from build123d import *

# Parameters (mm, degrees)
F1_DEPTH       = 22.86
F3_DEPTH       = 23.368
F5_DEPTH       = 45.72
F7_D           = 4.9784
F7_START       = 6.6163719
F7_CBORE_D     = 9.652
F7_CBORE_DEPTH = 2.54
F9_D           = 4.9784
F9_DEPTH       = 31.75
F9_CBORE_D     = 9.652
F9_CBORE_DEPTH = 12.7
F9_TIP         = 1.4956622529


with BuildPart() as f1:
    # F0 (on Front) → F1 (new body, symmetric)
    with BuildSketch(Plane.XZ):
        with BuildLine():
            ThreePointArc((-38.7916133821, 0), (-20.5036133821, 18.288), (-2.2156133821, 0))
            Line((-2.2156133821, 0), (10.4843866179, 0))
            Line((10.4843866179, 0), (26.3593866179, 0))
            Line((26.3593866179, 0), (42.2343866179, 0))
            Line((42.2343866179, 0), (49.8543866179, 0))
            Line((49.8543866179, 0), (49.8543866179, 19.05))
            Line((49.8543866179, 19.05), (-0.1977932308, 19.05))
            ThreePointArc((-0.1977932308, 19.05), (-3.2353429752, 19.6542062107), (-5.8104533064, 21.3748399243))
            Line((-5.8104533064, 21.3748399243), (-9.8356133821, 25.4))
            Line((-9.8356133821, 25.4), (-31.1716133821, 25.4))
            Line((-31.1716133821, 25.4), (-43.8716133821, 12.7))
            Line((-43.8716133821, 12.7), (-43.8716133821, 0))
            Line((-43.8716133821, 0), (-38.7916133821, 0))
        make_face()
        with BuildLine():
            ThreePointArc((-21.3164133821, -18.2699288493), (-33.7194264558, -12.640934649), (-38.7916133821, 0))
            Line((-38.7916133821, 0), (-43.8716133821, 0))
            Line((-43.8716133821, 0), (-43.8716133821, -12.7))
            Line((-43.8716133821, -12.7), (-31.1716133821, -25.4))
            Line((-31.1716133821, -25.4), (-21.3164133821, -25.4))
            Line((-21.3164133821, -25.4), (-21.3164133821, -18.2699288493))
        make_face()
        with BuildLine():
            ThreePointArc((-38.7916133821, 0), (-20.5036133821, 18.288), (-2.2156133821, 0))
            Line((-2.2156133821, 0), (10.4843866179, 0))
            Line((10.4843866179, 0), (26.3593866179, 0))
            Line((26.3593866179, 0), (42.2343866179, 0))
            Line((42.2343866179, 0), (49.8543866179, 0))
            Line((49.8543866179, 0), (49.8543866179, 19.05))
            Line((49.8543866179, 19.05), (-0.1977932308, 19.05))
            ThreePointArc((-0.1977932308, 19.05), (-3.2353429752, 19.6542062107), (-5.8104533064, 21.3748399243))
            Line((-5.8104533064, 21.3748399243), (-9.8356133821, 25.4))
            Line((-9.8356133821, 25.4), (-31.1716133821, 25.4))
            Line((-31.1716133821, 25.4), (-43.8716133821, 12.7))
            Line((-43.8716133821, 12.7), (-43.8716133821, 0))
            Line((-43.8716133821, 0), (-38.7916133821, 0))
        make_face()
        with BuildLine():
            Line((10.4843866179, 0), (-2.2156133821, 0))
            ThreePointArc((-2.2156133821, 0), (-7.2878003084, -12.640934649), (-19.6908133821, -18.2699288493))
            Line((-19.6908133821, -18.2699288493), (-19.6908133821, -25.4))
            Line((-19.6908133821, -25.4), (-9.8356133821, -25.4))
            Line((-9.8356133821, -25.4), (-5.8104533064, -21.3748399243))
            ThreePointArc((-5.8104533064, -21.3748399243), (-3.2353429752, -19.6542062107), (-0.1977932308, -19.05))
            Line((-0.1977932308, -19.05), (49.8543866179, -19.05))
            Line((49.8543866179, -19.05), (49.8543866179, 0))
            Line((49.8543866179, 0), (42.2343866179, 0))
            Line((42.2343866179, 0), (26.3593866179, 0))
            Line((26.3593866179, 0), (10.4843866179, 0))
        make_face()
    extrude(amount=F1_DEPTH, both=True)

    # F2 (on Top) → F3 (cut, symmetric)
    with BuildSketch(Plane.XY):
        with BuildLine():
            ThreePointArc((42.2135652835, -0.8128), (42.2291804306, -0.4065333221), (42.2343866179, 0))
            ThreePointArc((42.2343866179, 0), (42.2291804306, 0.4065333221), (42.2135652835, 0.8128))
            ThreePointArc((42.2135652835, 0.8128), (25.9528532958, 15.8697938127), (10.4843866179, 0))
            ThreePointArc((10.4843866179, 0), (25.9528532958, -15.8697938127), (42.2135652835, -0.8128))
        make_face()
        with BuildLine():
            ThreePointArc((42.2135652835, -0.8128), (42.2291804306, -0.4065333221), (42.2343866179, 0))
            ThreePointArc((42.2343866179, 0), (42.2291804306, 0.4065333221), (42.2135652835, 0.8128))
            ThreePointArc((42.2135652835, 0.8128), (25.9528532958, 15.8697938127), (10.4843866179, 0))
            ThreePointArc((10.4843866179, 0), (25.9528532958, -15.8697938127), (42.2135652835, -0.8128))
        make_face()
        with BuildLine():
            ThreePointArc((42.2135652835, 0.8128), (42.2291804306, 0.4065333221), (42.2343866179, 0))
            ThreePointArc((42.2343866179, 0), (42.2291804306, -0.4065333221), (42.2135652835, -0.8128))
            Line((42.2135652835, -0.8128), (49.8543866179, -0.8128))
            Line((49.8543866179, -0.8128), (49.8543866179, 0.8128))
            Line((49.8543866179, 0.8128), (42.2135652835, 0.8128))
        make_face()
        with BuildLine():
            ThreePointArc((42.2135652835, 0.8128), (42.2291804306, 0.4065333221), (42.2343866179, 0))
            ThreePointArc((42.2343866179, 0), (42.2291804306, -0.4065333221), (42.2135652835, -0.8128))
            Line((42.2135652835, -0.8128), (49.8543866179, -0.8128))
            Line((49.8543866179, -0.8128), (49.8543866179, 0.8128))
            Line((49.8543866179, 0.8128), (42.2135652835, 0.8128))
        make_face()
    extrude(amount=F3_DEPTH, both=True, mode=Mode.SUBTRACT)

    # F4 (on face) → F5 (cut)
    with BuildSketch(Plane.XY.offset(25.4)):
        with BuildLine():
            Line((7.7393313079, 19.05), (36.9442318174, 19.05))
            Line((36.9442318174, 19.05), (43.5606037016, 12.4336281158))
            Line((43.5606037016, 12.4336281158), (49.8543866179, 12.4336281158))
            Line((49.8543866179, 12.4336281158), (49.8543866179, 22.86))
            Line((49.8543866179, 22.86), (0.9593866179, 22.86))
            ThreePointArc((0.9593866179, 22.86), (3.8507663413, 20.0677479271), (7.7393313079, 19.05))
        make_face()
        with BuildLine():
            Line((43.5606037016, -12.4336281158), (36.9442318174, -19.05))
            Line((36.9442318174, -19.05), (7.7393313079, -19.05))
            ThreePointArc((7.7393313079, -19.05), (3.8507663413, -20.0677479271), (0.9593866179, -22.86))
            Line((0.9593866179, -22.86), (49.8543866179, -22.86))
            Line((49.8543866179, -22.86), (49.8543866179, -12.4336281158))
            Line((49.8543866179, -12.4336281158), (43.5606037016, -12.4336281158))
        make_face()
    extrude(amount=-F5_DEPTH, mode=Mode.SUBTRACT)

    # F7 (through all)
    # its depths count from where the whole tool has entered the part; down to there all is cleared
    with Locations(Plane.XZ.offset(19.05).offset(-F7_START)):
        with Locations((44.9775866179, 9.525), (44.9775866179, -9.525)):
            CounterBoreHole(F7_D / 2, F7_CBORE_D / 2, F7_CBORE_DEPTH)

    # F9
    with Locations(Plane(origin=(-43.8716133821, 0, 0), x_dir=(0, -1, 0), z_dir=(-1, 0, 0))):
        with Locations((13.335, 20.7645), (-13.335, 20.7645), (13.335, -20.7645), (-13.335, -20.7645)):
            CounterBoreHole(F9_D / 2, F9_CBORE_D / 2, F9_CBORE_DEPTH, depth=F9_DEPTH)
            with Locations((0, 0, -(F9_DEPTH + F9_TIP / 2))):  # 118° drill point
                Cone(0, F9_D / 2, F9_TIP, mode=Mode.SUBTRACT)


solid = f1.part
Verification items for the finished model (mm, model axes). A direction names the side the tool comes from. Round coordinates to 2 decimals unless told otherwise and drop trailing zeros. Order: outer loops, then holes, each group sorted by start corner. A loop starts at its lowest first (then second) coordinate and runs counter-clockwise, first axis right, second up. Notation, with made-up numbers: (-1, 11.5) -> (33, 11.5) arc R21 cw to (33, 38.5) -> close; hole circle Ø4 at (63, 20). An arc over 180 degrees is marked (long way). Put each result on its own line as item: value.
1) Section check B-B (x = 34). Record the cut outline in (y, z), then the cut area to 3 significant figures.
Final values:
outline: (-19.05, -19.05) -> (-13.92, -19.05) -> (-13.92, 19.05) -> (-19.05, 19.05) -> close; (13.92, -19.05) -> (19.05, -19.05) -> (19.05, 19.05) -> (13.92, 19.05) -> close
area: 391 mm^2
2) Mould release check, pull along X, two halves, no side actions. Record for faces 4 (the flat face through (-37, 22.86, -11)), 5 (the cylindrical face through (42.68, -5.29, 8.57)), 6 (the flat face through (39.564, -16.431, 0.267)), 7 (the conical face through (-10.886, -13.279, -20.336)): +X half, -X half, draft (parallel to the pull), parting line (faces both ways), or undercut.
Final values:
face 4: draft
face 5: undercut
face 6: +X half
face 7: -X half
3) Depth check by flat-ended pin: pin 1 (8 mm diameter, centred on x = 11.5, z = 9, fed in from -Y); pin 2 (12.5 mm diameter, centred on y = 13.34, z = -20.76, fed in from -X); pin 3 (6.5 mm diameter, centred on x = 44.98, z = -9.52, fed in from +Y). Enter the tip coordinate at first touch or a pass-through.
Final values:
pin 1: stops at y = -19.05
pin 2: stops at x = -42.06
pin 3: stops at y = 14.26
4) Set-up check for faces 1 (the cylindrical face through (-34.945, 13.528, 15.942)), 2 (the flat face through (14.1, -10.5, 19.05)), 3 (the flat face through (47, 12.434, 0)): record each of +Z, -Z, +X, -X, +Y, -Y from which the full face is reachable in a straight line by a thin tool's end or side.
Final values:
face 1: -X
face 2: +Z, +X, +Y, -Y
face 3: +Z, -Z, +X, +Y
5) Material ranges on line 1 (X direction, y = -5.5, z = -13); line 2 (X direction, y = 9.5, z = 3); line 3 (Z direction, x = -21.5, y = 8.5), recorded low to high.
Final values:
line 1: x = -43.57 to -33.37, -7.64 to 11.47, 41.25 to 49.85
line 2: x = -43.87 to -38.54, -2.46 to 13.64, 39.08 to 49.85
line 3: z = -25.4 to -18.26, 18.26 to 25.4
6) Section check A-A (y = 5). Give the number of separate pieces and of enclosed holes in the cut face, then the cut area to 3 significant figures.
Final values:
separate pieces: 2
enclosed holes: 2
area: 1,640 mm^2
